Here's how the part is built. I have some questions about the finished solid (model axes, mm). Face numbers are marked on the shaded views. A direction names the side the tool comes from. Give positions to 0.01 mm unless a question says otherwise; leave off trailing zeros. Order: outer loops, then holes, each group sorted by start corner. A loop starts at its lowest first (then second) coordinate and runs counter-clockwise, first axis right, second up. Notation, with made-up numbers: M -21,76 L 21,76 A18 cw 21,106 Z; hole C 34.5,89 d7. An arc over 180 degrees is marked long. Use one line per item in the form item = value.
from build123d import *

# Parameters (mm, degrees)
F1_DEPTH  = 2
F3_DEPTH  = 25
F4_R      = 1.5
F5_DEPTH  = 25
F7_DEPTH  = 12
F8_W      = 3
F8_H      = 9
F9_DEPTH  = 8
F10_W     = 2
F10_H     = 2
F11_DEPTH = 4
F12_R     = 1


with BuildPart() as f1:
    # F0 (on Top) → F1 (new body)
    with BuildSketch(Plane.XY):
        Polygon((-11.5, 8), (-11.5, 0), (11.5, 0), (11.5, 8), (1, 8), (1, 2), (-1, 2), (-1, 8), align=None)
    extrude(amount=F1_DEPTH)

    # F2 (on face) → F3 (cut)
    with BuildSketch(Plane.XY.offset(2)):
        Polygon((-1, 8), (-4, 8), (-1, 3), align=None)
        Polygon((1, 8), (1, 3), (4, 8), align=None)
    extrude(amount=-F3_DEPTH, mode=Mode.SUBTRACT)

    # F4 (on face) → F5 (cut)
    with BuildSketch(Plane.XY.offset(2)):
        with Locations((-8, 4)):
            Circle(F4_R)
        with Locations((8, 4)):
            Circle(F4_R)
    extrude(amount=-F5_DEPTH, mode=Mode.SUBTRACT)

    # F6 (on face) → F7 (join)
    with BuildSketch(Plane.XY.offset(2)):
        Polygon((-4, 8), (-5, 8), (-5, 0), (5, 0), (5, 8), (4, 8), (1, 3), (1, 2), (-1, 2), (-1, 3), align=None)
    extrude(amount=F7_DEPTH)

    # F8 (on face) → F9 (join)
    with BuildSketch(Plane(origin=(0, 8, 0), x_dir=(-1, 0, 0), z_dir=(0, 1, 0))):
        with Locations((2.5, 7)):
            Rectangle(F8_W, F8_H)
        with Locations((-2.5, 7)):
            Rectangle(F8_W, F8_H)
    extrude(amount=-F9_DEPTH)

    # F10 (on face) → F11 (join)
    with BuildSketch(Plane(origin=(0, 2, 0), x_dir=(-1, 0, 0), z_dir=(0, 1, 0))):
        with Locations((0, 7)):
            Rectangle(F10_W, F10_H)
    extrude(amount=F11_DEPTH)

    # F12
    f12_edges = [f1.edges().sort_by_distance(p)[0] for p in [
        (11.5, 8, 1),
        (11.5, 0, 1),
        (-11.5, 0, 1),
        (-11.5, 8, 1),
    ]]
    fillet(f12_edges, radius=F12_R)


solid = f1.part
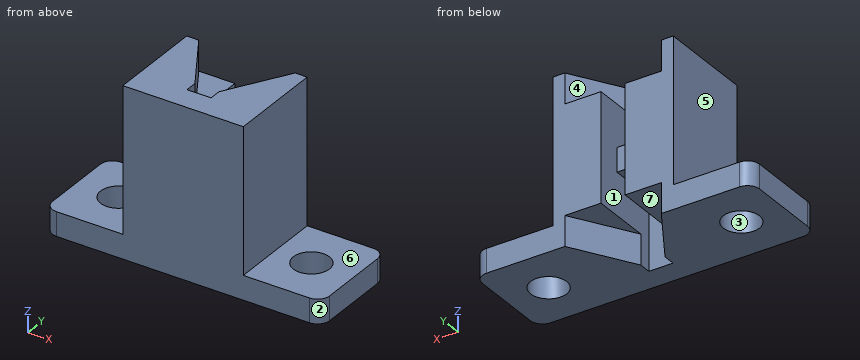
Q1. I want a section at A-A on x = -8. Write out the boundary of the cut face in (y, z), then the cut area to 3 significant figures.
Found:
outline = M 0,0 L 2.5,0 L 2.5,2 L 0,2 Z; M 5.5,0 L 8,0 L 8,2 L 5.5,2 Z
area = 10.0 mm²
Q2. On a 3-axis mill with a long thin cutter (end or side, diameter ignored), from which of +Z, -Z, +X, -X, +Y, -Y can I reach the whole of each face in a straight line? I mean the marked faces 4, 5, 6 and 7. Say none if no direction works.
Found:
face_4 = +Z, +Y
face_5 = +Z, -X, +Y, -Y
face_6 = +Z, +X, +Y, -Y
face_7 = -Z, +Y
Q3. I want a section at D-D on y = 1.25. Write out the boundary of the cut face in (x, z), then the cut area to 3 significant figures.
Found:
outline = M -11.5,0 L 11.5,0 L 11.5,2 L 5,2 L 5,14 L -5,14 L -5,2 L -11.5,2 Z
area = 166 mm²
Q4. I want a section at B-B on y = 4. State how many separate pieces and enclosed holes the cut face has, then the cut area to 3 significant figures.
Found:
separate_pieces = 3
enclosed_holes = 0
area = 124 mm²
Q5. I need wall thicknesses on L1, parallel to Y at x = 8, z = 1.65; L2, parallel to X at y = 2.25, z = 9.75; L3, parallel to Z at x = 2.75, y = 6.5. Which ranges of each line are inside material? Lowest first, please.
Found:
L1 = 0 to 2.5, 5.5 to 8
L2 = -5 to -1, 1 to 5
L3 = 2.5 to 11.5
Q6. I'm going to push flat-ended pins straight in: pin 1 Ø4 at (y, z) = (3, 9) entering from -X; pin 2 Ø0.6 at (x, z) = (0, 3.5) entering from +Y; pin 3 Ø1.8 at (x, y) = (-8, 4) entering from -Z; pin 4 Ø1.5 at (y, z) = (6.5, 12) entering from +X. Where does each tip first touch, or does it pass through?
Found:
pin_1 = -5
pin_2 = 2
pin_3 = through
pin_4 = 5
Q7. I want a section at C-C on z = 5.75. Write out the boundary of the cut face in (x, y).
Found:
outline = M -5,0 L 5,0 L 5,8 L 1,8 L 1,2 L -1,2 L -1,8 L -5,8 Z
Q8. Thinking about a two-plate mould opening in Y: for the marked faces 1, 2 and 3, which applies, +Y half, -Y half, draft (parallel to the pull), parting line (faces both ways), or undercut?
Found:
face_1 = draft
face_2 = -Y half
face_3 = undercut
